```python
from build123d import *

# Parameters (mm, degrees)
F0_W     = 100
F0_H     = 100
F1_DEPTH = 100
F2_T     = -3
F3_R     = 2
F4_DEPTH = 100.001


# Not quite as in the source:
# - a pattern or mirror of a feature is missing from the dataset's text; its kind, count and spacing are read off the source's solid


with BuildPart() as f1:
    # F0 (on Top) → F1 (new body)
    with BuildSketch(Plane.XY):
        Rectangle(F0_W, F0_H)
    extrude(amount=F1_DEPTH)

    # F2 (hollow: no face is removed)
    offset(amount=F2_T, mode=Mode.SUBTRACT)

    # F3 (on face) → F4 (cut, through all)
    with BuildSketch(Plane(origin=(-50, 0, 0), x_dir=(0, -1, 0), z_dir=(-1, 0, 0))):
        with Locations((0, 50)):
            Circle(F3_R)
    f4 = extrude(amount=-F4_DEPTH, mode=Mode.SUBTRACT)

    # F4_copies: F4 across plane
    add(f4.mirror(Plane(origin=(0, 0, 0), x_dir=(0.7071067812, 0.7071067812, 0), z_dir=(-0.7071067812, 0.7071067812, 0))), mode=Mode.SUBTRACT)


solid = f1.part
```
Input: part model. Units: mm. Frame: model coordinates. A direction names the side the tool comes from. Round coordinates to 2 decimals unless told otherwise and drop trailing zeros. Order: outer loops, then holes, each group sorted by start corner. A loop starts at its lowest first (then second) coordinate and runs counter-clockwise, first axis right, second up. Notation, with made-up numbers: (3.5, 32) - (25.5, 32) arc R23 cw to (25.5, 57) - close; hole circle Ø8 at (48, -33). An arc over 180 degrees is marked (long way). Answer in a Markdown table with one row per item.
Item 1: Mould query, pull axis Y, two halves, no side actions, for faces 3 (the flat face through (-1, 1, 97)), 4 (the flat face through (-1, 1, 3)), 5 (the flat face through (-1, -50, 38)), 6 (the flat face through (50, -1, 38)). Classes: released by +Y, released by -Y, zero draft, split by the parting line, or undercut.
Model answer:
| item | result |
|---|---|
| face 3 | undercut |
| face 4 | undercut |
| face 5 | released by -Y |
| face 6 | zero draft |
Item 2: Section query D-D (z = 21). Return the cut outline in (x, y), then the cut area to 3 significant figures.
Model answer:
| item | result |
|---|---|
| outline | (-50, -50) - (50, -50) - (50, 50) - (-50, 50) - close; hole (-47, -47) - (47, -47) - (47, 47) - (-47, 47) - close |
| area | 1,160 mm² |
Item 3: Reachability of faces 1 (the flat face through (-11, -47, 49)), 2 (the cylindrical face through (-48.521, -0.923, 48.226)) from +Z, -Z, +X, -X, +Y, -Y: full face, straight path, thin tool, end or side. Return the list, or none.
Model answer:
| item | result |
|---|---|
| face 1 | none |
| face 2 | +X, -X |
Item 4: Line query: line 1 (Y direction, x = 21, z = 55.5); line 2 (Z direction, x = -38.5, y = -32.5); line 3 (Z direction, x = 0, y = -48.7). Output: solid intervals per line, ascending.
Model answer:
| item | result |
|---|---|
| line 1 | y = -50 to -47, 47 to 50 |
| line 2 | z = 0 to 3, 97 to 100 |
| line 3 | z = 0 to 48, 52 to 100 |
Item 5: Section query B-B (z = 50). Return the cut outline in (x, y).
Model answer:
| item | result |
|---|---|
| outline | (-50, -50) - (-2, -50) - (-2, -47) - (-47, -47) - (-47, -2) - (-50, -2) - close; (-50, 2) - (-47, 2) - (-47, 47) - (-2, 47) - (-2, 50) - (-50, 50) - close; (2, -50) - (50, -50) - (50, -2) - (47, -2) - (47, -47) - (2, -47) - close; (2, 47) - (47, 47) - (47, 2) - (50, 2) - (50, 50) - (2, 50) - close |
Item 6: Section query A-A (x = 0). Return the cut outline in (y, z).
Model answer:
| item | result |
|---|---|
| outline | (-50, 0) - (50, 0) - (50, 48) - (47, 48) - (47, 3) - (-47, 3) - (-47, 48) - (-50, 48) - close; (-50, 52) - (-47, 52) - (-47, 97) - (47, 97) - (47, 52) - (50, 52) - (50, 100) - (-50, 100) - close |
